from build123d import *

# Parameters (mm, degrees)
ESQUISSE1_R                  = 13.7
ESQUISSE1_R_2                = 12.7
ESQUISSE3_W                  = 3.251730064
ESQUISSE3_H                  = 23.99378428
BOSS_EXTRU_1_DEPTH           = 4
R_P_TITION_CIRCULAIRE1_COUNT = 3


with BuildPart() as part:
    # Balayage1: sweep along a path in Esquisse2
    with BuildLine(Plane(origin=(0, 0, 0), x_dir=(1, 0, 0), z_dir=(0, 1, 0))) as balayage1_path:
        Line((0, 0), (26.30360969, 26.30360969))
    # Esquisse1 → Balayage1 (sweep)
    with BuildSketch(Plane.XY):
        Circle(ESQUISSE1_R)
        Circle(ESQUISSE1_R_2, mode=Mode.SUBTRACT)
    sweep(path=balayage1_path.line)

    # Esquisse3 → Boss.-Extru.1 (add)
    with BuildSketch(Plane.XY):
        with Locations((0, 11.99689214)):
            Rectangle(ESQUISSE3_W, ESQUISSE3_H)
    boss_extru_1 = extrude(amount=-BOSS_EXTRU_1_DEPTH)

    # Répétition circulaire1: Boss.-Extru.1 ×3 about axis
    r_p_tition_circulaire1_axis = Axis((0, 0, 0), (0, 0, 1))
    for i in range(1, R_P_TITION_CIRCULAIRE1_COUNT):
        add(boss_extru_1.rotate(r_p_tition_circulaire1_axis, i * 360 / R_P_TITION_CIRCULAIRE1_COUNT))


solid = part.part
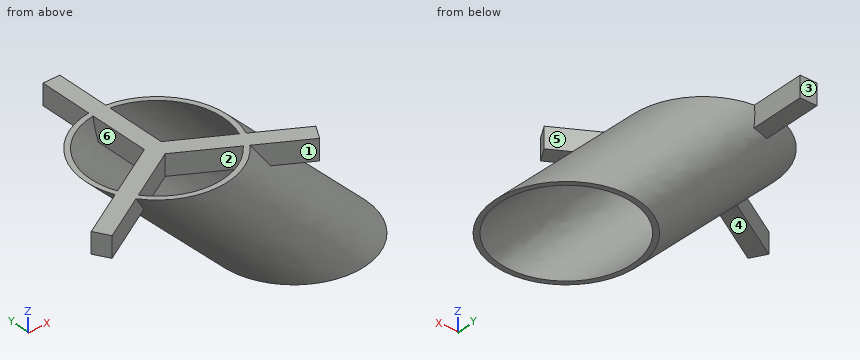
For this review, take the finished solid that the model builds, in its own axes (mm). Face numbers are marked on the shaded views. A direction names the side the tool comes from. Round coordinates to 2 decimals unless told otherwise and drop trailing zeros. Loops run counter-clockwise (first coordinate to the right, second up) from the corner with the lowest first, then second, coordinate; pieces in that order, holes last. Notation, with made-up numbers: (9, 37) - (58, 37) arc R14 cw to (58, 59) - close; hole circle Ø5 at (18, -39). An arc over 180 degrees is marked (long way). Use one line per item in the form item = value.
1) Clearance check with flat-ended pins moving along their axes: P1, Ø3, axis at y = -0.5, z = -22, coming from the +X side; P2, Ø10, axis at y = -6, z = -13.5, coming from the +X side; P3, Ø5, axis at y = -8.5, z = -22, coming from the -X side; P4, Ø5, axis at x = -5, y = 13.5, coming from the +Z side. State where each tip first meets the part, or that it passes through.
Solutions:
P1 = 37.19
P2 = 31.21
P3 = 8.21
P4 = 0
2) We need section A-A on z = -2.5. State how many separate pieces and enclosed holes the cut face has, then the cut area to 3 significant figures.
Solutions:
separate_pieces = 1
enclosed_holes = 3
area = 303 mm2
3) Wall thickness on probe 1 along X at (y, z) = (-0.5, -1.5); probe 2 along X at (y, z) = (10.5, -19); probe 3 along X at (y, z) = (2.5, -6.25): over which ranges is each line inside the solid? List them lowest first.
Solutions:
probe_1 = -12.19 to -11.19, -4.12 to 4.12, 14.19 to 15.19
probe_2 = 10.2 to 11.86, 26.14 to 27.8
probe_3 = -7.22 to -6.2, 18.7 to 19.72
4) Tool access review of the marked faces 1, 2 and 3: name each direction out of +Z, -Z, +X, -X, +Y, -Y from which nothing blocks a thin tool from reaching the whole face with its end or side.
Solutions:
face_1 = +Z, -Y
face_2 = none
face_3 = +Z, -Z, +X, -X, +Y
5) Mouldability with a two-part tool opening along X and no side actions: class the marked faces 4, 5 and 6 as pulls with the +X half, pulls with the -X half, needs draft (parallel to the pull), parting line crosses it, or undercut.
Solutions:
face_4 = needs draft
face_5 = pulls with the +X half
face_6 = undercut
6) We need section C-C on x = -15. Write out the cut boundary in (y, z), then the cut area to 3 significant figures.
Solutions:
outline = (-10.54, -4) - (-6.78, -4) - (-6.78, 0) - (-10.54, 0) - close
area = 15.0 mm2
